```python
from build123d import *

# Parameters (mm, degrees)
BOSS_EXTRUDE1_DEPTH        = 88.9
FLATTEN_BENDS1_START       = -88.9
FLATTEN_BENDS1_OUTLINE_W   = 1.98374
FLATTEN_BENDS1_OUTLINE_H   = 17.06626
FLATTEN_BENDS1_DEPTH       = 177.8
FLATTEN_BENDS1_2_OUTLINE_W = 16.324394327
FLATTEN_BENDS1_2_OUTLINE_H = 1.98374
FLATTEN_BENDS1_2_DEPTH     = 177.8
PROCESS_BENDS1_START       = -88.9
PROCESS_BENDS1_DEPTH       = 177.8
PROCESS_BENDS1_2_DEPTH     = 177.8
CUT_EXTRUDE1_DEPTH         = 137.077284035
F_8_0_199_DIAMETER_HOLE1_D = 5.0546
SKETCH14_R                 = 1.778
CUT_EXTRUDE2_DEPTH         = 1.98374


# Read off the part's stored shape, not the designer's step: Flatten-Bends1, Process-Bends1
with BuildPart() as part:
    # Sketch1 → Boss-Extrude1 (new, symmetric)
    with BuildSketch(Plane(origin=(0, 0, 0), x_dir=(1, 0, 0), z_dir=(0, 1, 0))):
        Polygon((0, 0), (0, 19.05), (1.98374, 19.05), (1.98374, 1.98374), (101.6, 1.98374), (101.6, 0), align=None)
    extrude(amount=BOSS_EXTRUDE1_DEPTH, both=True)

    # Flatten-Bends1 outline → Flatten-Bends1 (cut)
    with BuildSketch(Plane(origin=(0, 0, 0), x_dir=(1, 0, 0), z_dir=(0, 1, 0)).offset(FLATTEN_BENDS1_START)):
        with Locations((0.99187, 10.51687)):
            Rectangle(FLATTEN_BENDS1_OUTLINE_W, FLATTEN_BENDS1_OUTLINE_H)
    extrude(amount=FLATTEN_BENDS1_DEPTH, mode=Mode.SUBTRACT)

    # Flatten-Bends1 2 outline → Flatten-Bends1 2 (add)
    with BuildSketch(Plane(origin=(0, 0, 0), x_dir=(1, 0, 0), z_dir=(0, 1, 0)).offset(FLATTEN_BENDS1_START)):
        with Locations((-8.162197164, 0.99187)):
            Rectangle(FLATTEN_BENDS1_2_OUTLINE_W, FLATTEN_BENDS1_2_OUTLINE_H)
    extrude(amount=FLATTEN_BENDS1_2_DEPTH)

    # Process-Bends1 outline → Process-Bends1 (cut)
    with BuildSketch(Plane(origin=(0, 0, 0), x_dir=(1, 0, 0), z_dir=(0, 1, 0)).offset(PROCESS_BENDS1_START)):
        with BuildLine():
            ThreePointArc((2.72034, 0), (1.077712947, 0.551924431), (0.101624637, 1.98374))
            Line((0.101624637, 1.98374), (-16.324394327, 1.98374))
            Line((-16.324394327, 1.98374), (-16.324394327, 0))
            Line((-16.324394327, 0), (2.72034, 0))
        make_face()
    extrude(amount=PROCESS_BENDS1_DEPTH, mode=Mode.SUBTRACT)

    # Process-Bends1 2 outline → Process-Bends1 2 (add)
    with BuildSketch(Plane(origin=(0, 0, 0), x_dir=(1, 0, 0), z_dir=(0, 1, 0)).offset(PROCESS_BENDS1_START)):
        with BuildLine():
            Line((1.98374, 2.72034), (1.98374, 19.05))
            Line((1.98374, 19.05), (0, 19.05))
            Line((0, 19.05), (0, 2.72034))
            ThreePointArc((0, 2.72034), (0.025525919, 2.348551375), (0.101624637, 1.98374))
            Line((0.101624637, 1.98374), (2.72034, 1.98374))
            ThreePointArc((2.72034, 1.98374), (2.199485145, 2.199485145), (1.98374, 2.72034))
        make_face()
    extrude(amount=PROCESS_BENDS1_2_DEPTH)

    # Sketch6 → Cut-Extrude1 (cut, through all)
    with BuildSketch(Plane(origin=(0, 0, -1.98374), x_dir=(-1, 0, 0), z_dir=(0, 0, -1))):
        with BuildLine():
            Line((-92.60000004, -74.9115748), (-54.50000004, -74.9115748))
            ThreePointArc((-54.50000004, -74.9115748), (-52.31717484, -77.0944), (-54.50000004, -79.2772252))
            Line((-54.50000004, -79.2772252), (-92.60000004, -79.2772252))
            ThreePointArc((-92.60000004, -79.2772252), (-94.78282524, -77.0944), (-92.60000004, -74.9115748))
        make_face()
        with BuildLine():
            Line((-92.60000004, 85.0884252), (-54.50000004, 85.0884252))
            ThreePointArc((-54.50000004, 85.0884252), (-52.31717484, 82.9056), (-54.50000004, 80.7227748))
            Line((-54.50000004, 80.7227748), (-92.60000004, 80.7227748))
            ThreePointArc((-92.60000004, 80.7227748), (-94.78282524, 82.9056), (-92.60000004, 85.0884252))
        make_face()
        with BuildLine():
            Line((-30.2, 69.28846), (-17.5, 69.28846))
            ThreePointArc((-17.5, 69.28846), (-15.31814, 67.1066), (-17.5, 64.92474))
            Line((-17.5, 64.92474), (-30.2, 64.92474))
            ThreePointArc((-30.2, 64.92474), (-32.38186, 67.1066), (-30.2, 69.28846))
        make_face()
        with BuildLine():
            Line((-30.2, -80.71154), (-17.5, -80.71154))
            ThreePointArc((-17.5, -80.71154), (-15.31814, -82.8934), (-17.5, -85.07526))
            Line((-17.5, -85.07526), (-30.2, -85.07526))
            ThreePointArc((-30.2, -85.07526), (-32.38186, -82.8934), (-30.2, -80.71154))
        make_face()
        with BuildLine():
            Line((-23.9531652, 4.33846), (-53.41374, 4.33846))
            Line((-53.41374, 4.33846), (-53.41374, -66.3787496))
            ThreePointArc((-53.41374, -66.3787496), (-54.053074699, -67.922240101), (-55.5965652, -68.5615748))
            Line((-55.5965652, -68.5615748), (-80.3671748, -68.5615748))
            ThreePointArc((-80.3671748, -68.5615748), (-81.910665301, -67.922240101), (-82.55, -66.3787496))
            Line((-82.55, -66.3787496), (-82.55, 56.3919148))
            ThreePointArc((-82.55, 56.3919148), (-81.910665301, 57.935405301), (-80.3671748, 58.57474))
            Line((-80.3671748, 58.57474), (-23.9531652, 58.57474))
            ThreePointArc((-23.9531652, 58.57474), (-22.409674699, 57.935405301), (-21.77034, 56.3919148))
            Line((-21.77034, 56.3919148), (-21.77034, 6.5212852))
            ThreePointArc((-21.77034, 6.5212852), (-22.409674699, 4.977794699), (-23.9531652, 4.33846))
        make_face()
    extrude(amount=-CUT_EXTRUDE1_DEPTH, mode=Mode.SUBTRACT)

    # #8 (0.199) Diameter Hole1 (through all)
    with Locations(Plane(origin=(1.98374, 0, 0), x_dir=(0, 0, -1), z_dir=(1, 0, 0))):
        with Locations((12.7, 69.85), (12.7, -76.2)):
            Hole(F_8_0_199_DIAMETER_HOLE1_D / 2)

    # Sketch14 → Cut-Extrude2 (cut)
    with BuildSketch(Plane.XY):
        with Locations((10.56374, -5.51154)):
            Circle(SKETCH14_R)
        with Locations((43.56374, -5.51154)):
            Circle(SKETCH14_R)
        with Locations((10.56374, -64.51154)):
            Circle(SKETCH14_R)
        with Locations((43.56374, -64.51154)):
            Circle(SKETCH14_R)
    extrude(amount=-CUT_EXTRUDE2_DEPTH, mode=Mode.SUBTRACT)


solid = part.part
```
Can you work these out from the model? Positions are in its coordinate system, mm. A direction names the side the tool comes from. Give positions to 0.01 mm unless a question says otherwise; leave off trailing zeros. Loops run counter-clockwise (first coordinate to the right, second up) from the corner with the lowest first, then second, coordinate; pieces in that order, holes last. Notation, with made-up numbers: M 54,3.25 L 80,3.25 A14 cw 80,22.25 Z; hole C 37.5,72.5 d9. An arc over 180 degrees is marked long. Answer in a Markdown table with one row per item.
1. Which directions (+Z, -Z, +X, -X, +Y, -Y) give clear straight access to the entire face, cutting with the end or side of a thin tool? Please do faces 5 (the cylindrical face through (9.15, -6.59, -0.98)), 6 (the flat face through (51, -1, -1.984)).
Taken from the geometry:
| item | result |
|---|---|
| face 5 | +Z, -Z |
| face 6 | -Z, +X, +Y, -Y |
2. For pin 1 Ø10 at (x, z) = (48.5, -9.5) entering from -Y; pin 2 Ø1 at (x, y) = (56.5, -70) entering from -Z; pin 3 Ø1.5 at (y, z) = (-10.5, -8) entering from +X, each with a flat end and sliding along its axis, tell me the tip position at first contact or that it passes through.
Taken from the geometry:
| item | result |
|---|---|
| pin 1 | passes through |
| pin 2 | stops at z = -1.98 |
| pin 3 | stops at x = 1.98 |
3. Thinking about a two-plate mould opening in X: for faces 1 (the flat face through (1.984, -1, -11)), 2 (the flat face through (0, -1, -11)), 3 (the cylindrical face through (45.206, -65.193, -0.978)), 4 (the flat face through (39.3, 88.9, -1.8)), which applies, released by +X, released by -X, zero draft, split by the parting line, or undercut?
Taken from the geometry:
| item | result |
|---|---|
| face 1 | released by +X |
| face 2 | released by -X |
| face 3 | undercut |
| face 4 | zero draft |
4. Suppose I cut it at D-D on y = 62.5. Write out the boundary of the cut face in (x, z).
Taken from the geometry:
| item | result |
|---|---|
| outline | M 0,-19.05 L 1.98,-19.05 L 1.98,-2.72 A0.74 cw 2.72,-1.98 L 101.6,-1.98 L 101.6,0 L 2.72,0 A2.72 ccw 0,-2.72 Z |
5. Suppose I cut it at B-B on x = 38. Write out the boundary of the cut face in (y, z), plus the area to 3 significant figures.
Taken from the geometry:
| item | result |
|---|---|
| outline | M -88.9,-1.98 L 4.34,-1.98 L 4.34,0 L -88.9,0 Z; M 58.57,-1.98 L 88.9,-1.98 L 88.9,0 L 58.57,0 Z |
| area | 245 mm² |
6. Suppose I cut it at C-C on z = -12.7. Write out the boundary of the cut face in (x, y), plus the area to 3 significant figures.
Taken from the geometry:
| item | result |
|---|---|
| outline | M 0,-88.9 L 1.98,-88.9 L 1.98,-78.73 L 0,-78.73 Z; M 0,-73.67 L 1.98,-73.67 L 1.98,67.32 L 0,67.32 Z; M 0,72.38 L 1.98,72.38 L 1.98,88.9 L 0,88.9 Z |
| area | 333 mm² |
7. Suppose I cut it at A-A on y = 31.5. Write out the boundary of the cut face in (x, z).
Taken from the geometry:
| item | result |
|---|---|
| outline | M 0,-19.05 L 1.98,-19.05 L 1.98,-2.72 A0.74 cw 2.72,-1.98 L 21.77,-1.98 L 21.77,0 L 2.72,0 A2.72 ccw 0,-2.72 Z; M 82.55,-1.98 L 101.6,-1.98 L 101.6,0 L 82.55,0 Z |
8. If I drill on line 1 along Z through (x, y) = (15, -78.5); line 2 along X through (y, z) = (72, -2.5); line 3 along X through (y, z) = (6.5, -1.5), over which ranges is the centre line in solid material (lowest first)?
Taken from the geometry:
| item | result |
|---|---|
| line 1 | z = -1.98 to 0 |
| line 2 | x = 0.01 to 2.02 |
| line 3 | x = 0.29 to 21.77, 82.55 to 101.6 |
